Read the model definition and answer for the solid it produces. Units are mm, in the model's axes. Give positions to 0.01 mm unless a question says otherwise; leave off trailing zeros. Write each loop counter-clockwise with the first axis right and the second up, starting at its lowest first coordinate (ties: lowest second). Pieces come first, ordered by that corner, then holes. Notation, with made-up numbers: M 18,73 L 69,73 A12 ccw 69,92 Z; hole C 37,9.5 d9. An arc over 180 degrees is marked long. Use a Markdown table: item, result. Add a question column.
Item 1: A cutting plane is placed at B-B on x = 0. Determine the outline of the cut face in (y, z), then the cut area to 3 significant figures.
Item 2: Given P1, Ø3.5, axis at x = 42, z = 6, coming from the +Y side; P2, Ø4, axis at x = 41, y = -0.5, coming from the +Z side; P3, Ø4.5, axis at x = 42.5, z = 4, coming from the -Y side, each flat-ended and moving along its own axis, determine where each tip first touches the part or whether it passes through.
Item 3: A cutting plane is placed at A-A on y = 0. Determine the outline of the cut face in (x, z), then the cut area to 3 significant figures.
Item 4: A cutting plane is placed at C-C on z = 6. Determine the outline of the cut face in (x, y).
Item 5: Consider probe 1 along Y at (x, z) = (0, 3); probe 2 along X at (y, z) = (119, 74.5); probe 3 along Z at (x, y) = (36, -2.5). Determine where each line is inside the solid, lowest interval first. Write a range as [from, to].
Item 6: A cutting plane is placed at D-D on x = -24. Determine the outline of the cut face in (y, z).
from build123d import *

# Parameters (mm, degrees)
BOX_W             = 10
BOX_H             = 10
BOX_DEPTH         = 10
BOX001_W          = 10
BOX001_H          = 240
BOX001_DEPTH      = 80
CYLINDER001_R     = 36
CYLINDER001_DEPTH = 10
CYLINDER_R        = 40
CYLINDER_DEPTH    = 10


with BuildPart() as cube:
    # Box → Box (new body)
    with BuildSketch(Plane(origin=(38, -5, 0), x_dir=(1, 0, 0), z_dir=(0, 0, 1))):
        with Locations((5, 5)):
            Rectangle(BOX_W, BOX_H)
    extrude(amount=BOX_DEPTH)


with BuildPart() as cube001:
    # Box001 → Box001 (new body)
    with BuildSketch(Plane(origin=(44, -108, 0), x_dir=(1, 0, 0), z_dir=(0, 0, 1))):
        with Locations((5, 120)):
            Rectangle(BOX001_W, BOX001_H)
    extrude(amount=BOX001_DEPTH)


with BuildPart() as cylinder001:
    # Cylinder001 → Cylinder001 (new body)
    with BuildSketch(Plane.XY):
        Circle(CYLINDER001_R)
    extrude(amount=CYLINDER001_DEPTH)


with BuildPart() as fusion:
    # Cylinder → Cylinder (new body)
    with BuildSketch(Plane.XY):
        Circle(CYLINDER_R)
    extrude(amount=CYLINDER_DEPTH)

    # Cut: cut Cylinder001
    add(cylinder001.part, mode=Mode.SUBTRACT)

    # Fusion: union Cube, Cube001
    add(cube.part)
    add(cube001.part)


solid = fusion.part
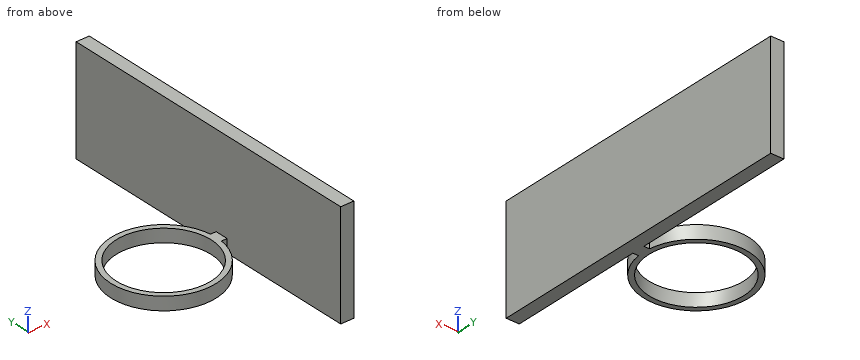
Filled in:
| question | item | result |
|---|---|---|
| 1 | outline | M -40,0 L -36,0 L -36,10 L -40,10 Z; M 36,0 L 40,0 L 40,10 L 36,10 Z |
| 1 | area | 80.0 mm² |
| 2 | P1 | y = 5 |
| 2 | P2 | z = 10 |
| 2 | P3 | y = -108 |
| 3 | outline | M -40,0 L -36,0 L -36,10 L -40,10 Z; M 36,0 L 54,0 L 54,80 L 44,80 L 44,10 L 36,10 Z |
| 3 | area | 920 mm² |
| 4 | outline | M 39.69,-5 L 44,-5 L 44,-108 L 54,-108 L 54,132 L 44,132 L 44,5 L 39.69,5 A40 ccw long Z; hole C 0,0 d72 |
| 5 | probe 1 | [-40, -36], [36, 40] |
| 5 | probe 2 | [44, 54] |
| 5 | probe 3 | [0, 10] |
| 6 | outline | M -32,0 L -26.83,0 L -26.83,10 L -32,10 Z; M 26.83,0 L 32,0 L 32,10 L 26.83,10 Z |
